Check sheet for the modelled part. Datum: model origin and axes. Units: mm. A direction names the side the tool comes from. Give positions to 0.01 mm unless a question says otherwise; leave off trailing zeros. Loops run counter-clockwise (first coordinate to the right, second up) from the corner with the lowest first, then second, coordinate; pieces in that order, holes last. Notation, with made-up numbers: (48, 5.5) -> (98, 5.5) arc R27 ccw to (98, 41.5) -> close; hole circle Ø5 at (77.25, 40.25). An arc over 180 degrees is marked (long way). Write each question's results on one line, items separated by ' | '. Start each with the question number.
Item 1: Gauge pin test, flat ends, axial feed: pin 1 Ø1.7 at (y, z) = (0.5, -66.5) entering from -X; pin 2 Ø2 at (x, z) = (-12.5, -45.5) entering from +Y. Record the tip position at first contact, or that the pin passes through.
Item 2: Cross-section at C-C on z = -54. Enter the section's corners in (x, y), then the cut area to 3 significant figures.
Item 3: Cross-section at B-B on x = 5. Enter the section's corners in (y, z).
Item 4: Mould release check, pull along Y, two halves, no side actions. Record for faces 3 (the face through (-16, 6, -18.849)), 4 (the face through (-25.86, 7.45, -83.53)), 5 (the face through (-31.44, 9.28, -18.04)): pulls with the +Y half, pulls with the -Y half, needs draft (parallel to the pull), parting line crosses it, or undercut.
Item 5: Access from +Z, -Z, +X, -X, +Y, -Y to the whole of each face (thin tool, end or side, straight path). Record for faces 1 (the face through (-8, 1.588, -50)), 2 (the face through (-9, 0, -51)).
Item 6: Cross-section at D-D on y = 9.5. Enter the section's corners in (x, z).
Item 7: Cross-section at A-A on y = 5.5. Enter the section's corners in (x, z), then the cut area to 3 significant figures.
Item 8: Scan lines: line 1 along Z through (x, y) = (-16.5, 11); line 2 along Y through (x, z) = (-16, -57.5). Record each from-to range of solid material in increasing order.
from build123d import *

# Parameters (mm, degrees)
SKETCH2_W           = 33.3375
SKETCH2_H           = 67.071875
BOSS_EXTRUDE1_DEPTH = 1.5875
SKETCH3_R           = 0.79375
BOSS_EXTRUDE2_DEPTH = 67.071875
SKETCH4_W           = 63.896875
SKETCH4_H           = 12.7
CUT_EXTRUDE1_DEPTH  = 40.6875


with BuildPart() as part:
    # Sketch2 → Boss-Extrude1 (new body)
    with BuildSketch(Plane(origin=(0, 0, 0), x_dir=(1, 0, 0), z_dir=(0, 1, 0))):
        with Locations((-8.563888889, 50.797800926)):
            Rectangle(SKETCH2_W, SKETCH2_H)
    extrude(amount=BOSS_EXTRUDE1_DEPTH)

    # Sketch3 → Boss-Extrude2 (add)
    with BuildSketch(Plane.XY.offset(-17.261863426)):
        with BuildLine():
            Line((-25.232638889, 1.5875), (8.104861111, 1.5875))
            Line((8.104861111, 1.5875), (-22.898284403, 13.84286105))
            ThreePointArc((-22.898284403, 13.84286105), (-31.470488786, 9.125661885), (-25.232638889, 1.5875))
        make_face()
        with Locations((-25.232638889, 7.9375)):
            Circle(SKETCH3_R, mode=Mode.SUBTRACT)
    extrude(amount=-BOSS_EXTRUDE2_DEPTH)

    # Sketch4 → Cut-Extrude1 (cut, through all)
    with BuildSketch(Plane(origin=(8.104861111, 0, 0), x_dir=(0, 0, -1), z_dir=(1, 0, 0))):
        with Locations((50.797800926, 7.9375)):
            Rectangle(SKETCH4_W, SKETCH4_H)
    extrude(amount=-CUT_EXTRUDE1_DEPTH, mode=Mode.SUBTRACT)


solid = part.part
Answer sheet:
1) pin 1: stops at x = -25.23 | pin 2: stops at y = 1.59
2) outline: (-25.23, 0) -> (8.1, 0) -> (8.1, 1.59) -> (-25.23, 1.59) -> close | area: 52.9 mm²
3) outline: (0, -84.33) -> (2.81, -84.33) -> (2.81, -82.75) -> (1.59, -82.75) -> (1.59, -18.85) -> (2.81, -18.85) -> (2.81, -17.26) -> (0, -17.26) -> close
4) face 3: needs draft | face 4: undercut | face 5: parting line crosses it
5) face 1: +X, -X, +Y | face 2: +Z, -Z, +X, -X, -Y
6) outline: (-31.39, -84.33) -> (-11.91, -84.33) -> (-11.91, -82.75) -> (-31.39, -82.75) -> close; (-31.39, -18.85) -> (-11.91, -18.85) -> (-11.91, -17.26) -> (-31.39, -17.26) -> close
7) outline: (-31.1, -84.33) -> (-1.79, -84.33) -> (-1.79, -82.75) -> (-31.1, -82.75) -> close; (-31.1, -18.85) -> (-1.79, -18.85) -> (-1.79, -17.26) -> (-31.1, -17.26) -> close | area: 93.0 mm²
8) line 1: z = -84.33 to -82.75, -18.85 to -17.26 | line 2: y = 0 to 1.59
